Autodesk Inventor part; units mm, degrees
ref_plane "YZ Plane" through (0, 0, 0) normal (1, 0, 0) x (0, 1, 0)
ref_plane "XZ Plane" through (0, 0, 0) normal (0, 1, 0) x (-1, 0, 0)
ref_plane "XY Plane" through (0, 0, 0) normal (0, 0, 1) x (1, 0, 0)
sketch "Sketch1" plane through (0, 0, 0) normal (0, 1, 0) x (-1, 0, 0)
  line L0 (23.5034, -42.4981) -> (-1.8966, -42.4981)
  line L1 (-1.8966, -42.4981) -> (-1.8966, 770.3019)
  line L2 (-1.8966, 770.3019) -> (23.5034, 770.3019)
  line L3 (23.5034, 770.3019) -> (23.5034, -42.4981)
  line L4 (20.3284, -39.3231) -> (1.2784, -39.3231)
  line L5 (1.2784, -39.3231) -> (1.2784, 767.1269)
  line L6 (1.2784, 767.1269) -> (20.3284, 767.1269)
  line L7 (20.3284, 767.1269) -> (20.3284, -39.3231)
  point P0 (0, 0)
  dimension "d0" = 25.4
  dimension "d1" = 812.8
  dimension "d2" = 3.175
ref_plane "Work Plane3" through (0, 0, 0) normal (0, -1, 0) x (1, 0, 0)
sketch "Sketch2" plane through (0, 0, 0) normal (0, -1, 0) x (1, 0, 0)
  line L0 (-1.2784, -39.3231) -> (-20.3284, -39.3231)
  line L1 (-20.3284, -39.3231) -> (-20.3284, 767.1269)
  line L2 (-1.2784, -39.3231) -> (-20.3284, -39.3231)
  line L3 (-20.3284, -39.3231) -> (-20.3284, 767.1269)
  line L4 (-20.3284, 767.1269) -> (-1.2784, 767.1269)
  line L5 (-1.2784, 767.1269) -> (-1.2784, -39.3231)
  point P0 (0, 0)
extrude "Extrusion3" add sketch "Sketch2" against normal blind 3.175
extrude "Extrusion5" add sketch "Sketch1" along normal blind 50.8
sketch "Sketch4" plane through (-23.5034, 0, 770.3019) normal (0, 0, 1) x (1, 0, 0)
  line L0 (0, 50.8) -> (25.4, 50.8)
  line L1 (0, 50.8) -> (3.175, 50.8)
  line L2 (3.175, 50.8) -> (25.4, 50.8)
  line L3 (25.4, 50.8) -> (22.225, 50.8)
  line L4 (22.225, 3.175) -> (22.225, 50.8)
  line L5 (3.175, 50.8) -> (22.225, 50.8)
  line L6 (22.225, 50.8) -> (22.225, 3.175)
  line L7 (22.225, 3.175) -> (3.175, 3.175)
  line L8 (3.175, 3.175) -> (3.175, 50.8)
  point P0 (23.5034, 0)
  point P1 (22.225, 0)
  dimension "d13" = 3.175
  dimension "d14" = 3.175
extrude "Extrusion6" cut sketch "Sketch4" against normal blind 1016
sketch "Sketch5" plane through (1.8966, 0, 770.3019) normal (1, 0, 0) x (0, 0, -1)
  line L0 (0, 0) -> (19.05, 0)
  line L1 (19.05, 0) -> (19.05, 25.4)
  line L2 (19.05, 25.4) -> (0, 25.4)
  line L3 (0, 25.4) -> (0, 0)
  circle A0 centre (19.05, 25.4) radius 14.2875
  line L4 (19.05, 25.4) -> (76.2, 25.4)
  circle A1 centre (76.2, 25.4) radius 14.2875
  line L5 (76.2, 25.4) -> (107.95, 25.4)
  circle A2 centre (107.95, 25.4) radius 14.2875
  point P0 (770.3019, 0)
  dimension "d17" = 19.05
  dimension "d18" = 25.4
  dimension "d19" = 28.575
  dimension "d22" = 57.15
  dimension "d23" = 28.575
  dimension "d26" = 31.75
  dimension "d27" = 28.575
extrude "Extrusion10" cut sketch "Sketch5" against normal blind 50.8 contours A2 | A1 L5 L4 | L4 L5 A1 | A0 L2 L1 | L1 L4 A0 | A0 L4 L2
sketch "Sketch6" plane through (1.8966, 0, 770.3019) normal (1, 0, 0) x (0, 0, -1)
  line L0 (812.8, 0) -> (812.8, 50.8)
  line L1 (812.8, 25.4) -> (781.05, 25.4)
  circle A0 centre (781.05, 25.4) radius 14.2875
  point P0 (770.3019, 0)
  dimension "d32" = 31.75
  dimension "d33" = 28.575
extrude "Extrusion11" cut sketch "Sketch6" against normal blind 76.2
properties part number "36in Aluminum Channel"
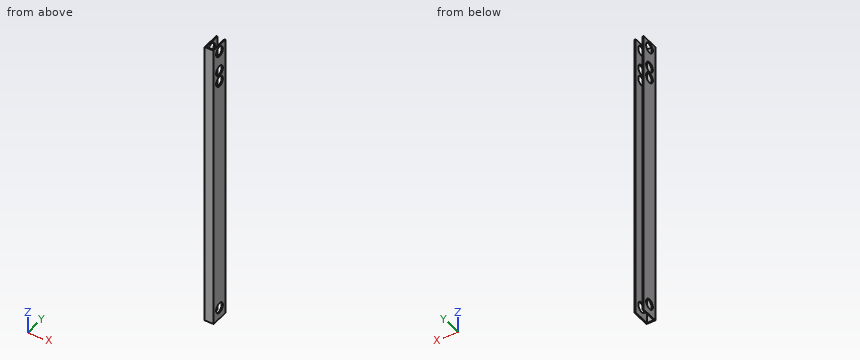
For this review, take the finished solid that the model builds, in its own axes (mm). Round coordinates to 2 decimals unless told otherwise and drop trailing zeros. Order: outer loops, then holes, each group sorted by start corner. A loop starts at its lowest first (then second) coordinate and runs counter-clockwise, first axis right, second up. Notation, with made-up numbers: (79, 3) -> (116, 3) arc R5 cw to (116, 11) -> close; hole circle Ø10 at (7.5, 0.25). An arc over 180 degrees is marked (long way). Put each result on its own line as item: value.
Q1. Add section A-A on z = 194.5. Write out the cut boundary in (x, y) (3 decimals).
Check result:
outline: (-23.503, 0) -> (1.897, 0) -> (1.897, 50.8) -> (-1.278, 50.8) -> (-1.278, 3.175) -> (-20.328, 3.175) -> (-20.328, 50.8) -> (-23.503, 50.8) -> close
Q2. For probe 1 along Z at (x, y) = (1, 25.5); probe 2 along X at (y, z) = (45.5, 38); probe 3 along Y at (x, z) = (-20.25, 453) (3 decimals), list the stretches that pass through material, from the lowest coordinate up. Write a range as [from, to].
Check result:
probe 1: [-42.5, -25.04], [3.54, 648.06], [676.64, 679.81], [708.39, 736.96], [765.54, 770.3]
probe 2: [-23.5, -20.33], [-1.28, 1.9]
probe 3: [0, 3.175]
Q3. Add section B-B on y = 25.4. State how many separate pieces and enclosed holes the cut face has, plus the area to 3 significant figures.
Check result:
separate pieces: 10
enclosed holes: 0
area: 4,440 mm2
Q4. Insertion check: pin 1 Ø3 at (x, z) = (-6, 479.5) entering from +Y (3 decimals); pin 2 Ø23 at (y, z) = (25.4, 662.35) entering from -X. Each pin has a flat end and moves straight along its axis. Give the tip position at first contact, or say it passes through.
Check result:
pin 1: y = 3.175
pin 2: through
Q5. Add section C-C on x = -12. Write out the cut boundary in (y, z) (3 decimals), plus the area to 3 significant figures.
Check result:
outline: (0, -42.498) -> (3.175, -42.498) -> (3.175, 770.302) -> (0, 770.302) -> close
area: 2,580 mm2
